Check sheet for the modelled part. Datum: model origin and axes. Units: mm. Give positions to 0.01 mm unless a question says otherwise; leave off trailing zeros. Order: outer loops, then holes, each group sorted by start corner. A loop starts at its lowest first (then second) coordinate and runs counter-clockwise, first axis right, second up. Notation, with made-up numbers: M 9,78 L 21,78 A12 ccw 21,99 Z; hole C 2.25,74 d6. An arc over 180 degrees is marked long. One line per question, with ' | ' between items. Start each with the question number.
```python
from build123d import *

# Parameters (mm, degrees)
F0_W      = 24
F0_H      = 9
F1_DEPTH  = 4
F2_W      = 8
F2_H      = 9
F2_R      = 3
F3_DEPTH  = 4
F4_W      = 8
F4_H      = 9
F4_R      = 3
F5_DEPTH  = 4
F6_W      = 14.751910232
F6_H      = 8.5369339213
F7_DEPTH  = 1000
F8_W      = 10
F8_H      = 4
F9_DEPTH  = 20
F10_DEPTH = 20
F11_R     = 1.9919096681
F12_DEPTH = 50


with BuildPart() as f1:
    # F0 (on Right) → F1 (new body, symmetric)
    with BuildSketch(Plane.YZ):
        Rectangle(F0_W, F0_H)
    extrude(amount=F1_DEPTH, both=True)

    # F2 (on face) → F3 (cut)
    with BuildSketch(Plane.XZ.offset(12)):
        Rectangle(F2_W, F2_H)
        Circle(F2_R, mode=Mode.SUBTRACT)
    extrude(amount=-F3_DEPTH, mode=Mode.SUBTRACT)

    # F4 (on face) → F5 (cut)
    with BuildSketch(Plane(origin=(0, 12, 0), x_dir=(-1, 0, 0), z_dir=(0, 1, 0))):
        Rectangle(F4_W, F4_H)
        Circle(F4_R, mode=Mode.SUBTRACT)
    extrude(amount=-F5_DEPTH, mode=Mode.SUBTRACT)

    # F6 (on face) → F7 (join)
    with BuildSketch(Plane.YZ.offset(4)):
        Rectangle(F6_W, F6_H)
    extrude(amount=F7_DEPTH)

    # F8 (on face) → F9 (join)
    with BuildSketch(Plane(origin=(0, 0, -4.2684669606), x_dir=(1, 0, 0), z_dir=(0, 0, -1))):
        with Locations((410.2546322346, 5.375955116)):
            Rectangle(F8_W, F8_H)
    extrude(amount=F9_DEPTH)

    # F8 (on face) → F10 (join)
    with BuildSketch(Plane(origin=(0, 0, -4.2684669606), x_dir=(1, 0, 0), z_dir=(0, 0, -1))):
        with Locations((410.2546322346, -5.375955116)):
            Rectangle(F8_W, F8_H)
    extrude(amount=F10_DEPTH)

    # F11 (on face) → F12 (cut)
    with BuildSketch(Plane.XZ.offset(7.375955116)):
        with Locations((410.2546322346, -20.4669394419)):
            Circle(F11_R)
    extrude(amount=-F12_DEPTH, mode=Mode.SUBTRACT)


solid = f1.part
```
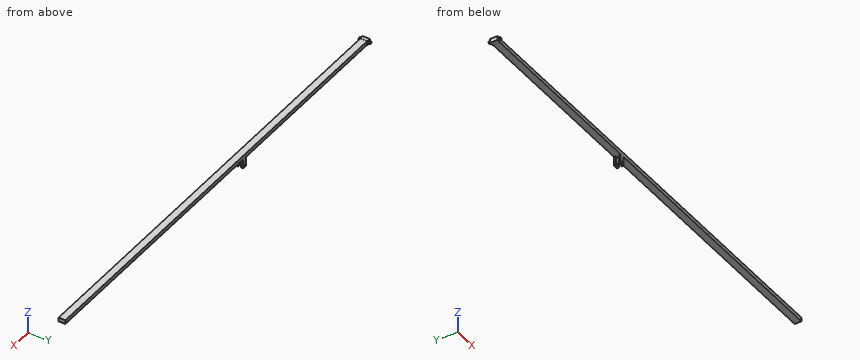
Item 1: Section check A-A, the plane z = -11. Record the cut outline in (x, y).
Item 2: Go/stop test with flat-tipped pins: P1, Ø8, axis at x = 410, z = -18.5, coming from the -Y side; P2, Ø11, axis at x = 409, z = -10.5, coming from the +Y side; P3, Ø6, axis at x = 894, y = -8.5, coming from the +Z side; P4, Ø3, axis at y = 1, z = -14, coming from the -X side. Record where each tip stops, or that it passes through.
Item 3: Section check B-B, the plane x = 78.5. Record the cut outline in (y, z).
Item 4: Scan lines: probe 1 along Y at (x, z) = (371, -3.5); probe 2 along Z at (x, y) = (821.5, -3.25); probe 3 along X at (y, z) = (6.25, -11.75). Record each from-to range of solid material in increasing order. Write a range as [from, to].
Reported:
1) outline: M 405.25,-7.38 L 415.25,-7.38 L 415.25,-3.38 L 405.25,-3.38 Z; M 405.25,3.38 L 415.25,3.38 L 415.25,7.38 L 405.25,7.38 Z
2) P1: stops at y = -7.38 | P2: stops at y = 7.38 | P3: stops at z = 4.27 | P4: passes through
3) outline: M -7.38,-4.27 L 7.38,-4.27 L 7.38,4.27 L -7.38,4.27 Z
4) probe 1: y = [-7.38, 7.38] | probe 2: z = [-4.27, 4.27] | probe 3: x = [405.25, 415.25]
